Job drawing, mm, ordinate dimensions from the low corner. One solid piece. Round coordinates to 2 decimals unless told otherwise and drop trailing zeros. Write each loop counter-clockwise with the first axis right and the second up, starting at its lowest first coordinate (ties: lowest second). Pieces come first, ordered by that corner, then holes. Notation, with made-up numbers: (-2, 52) - (30, 52) arc R12 ccw to (30, 63) - close; hole circle Ø11 at (11, 2.25). An arc over 180 degrees is marked (long way). Write each question's results on one line, items separated by ' | '.
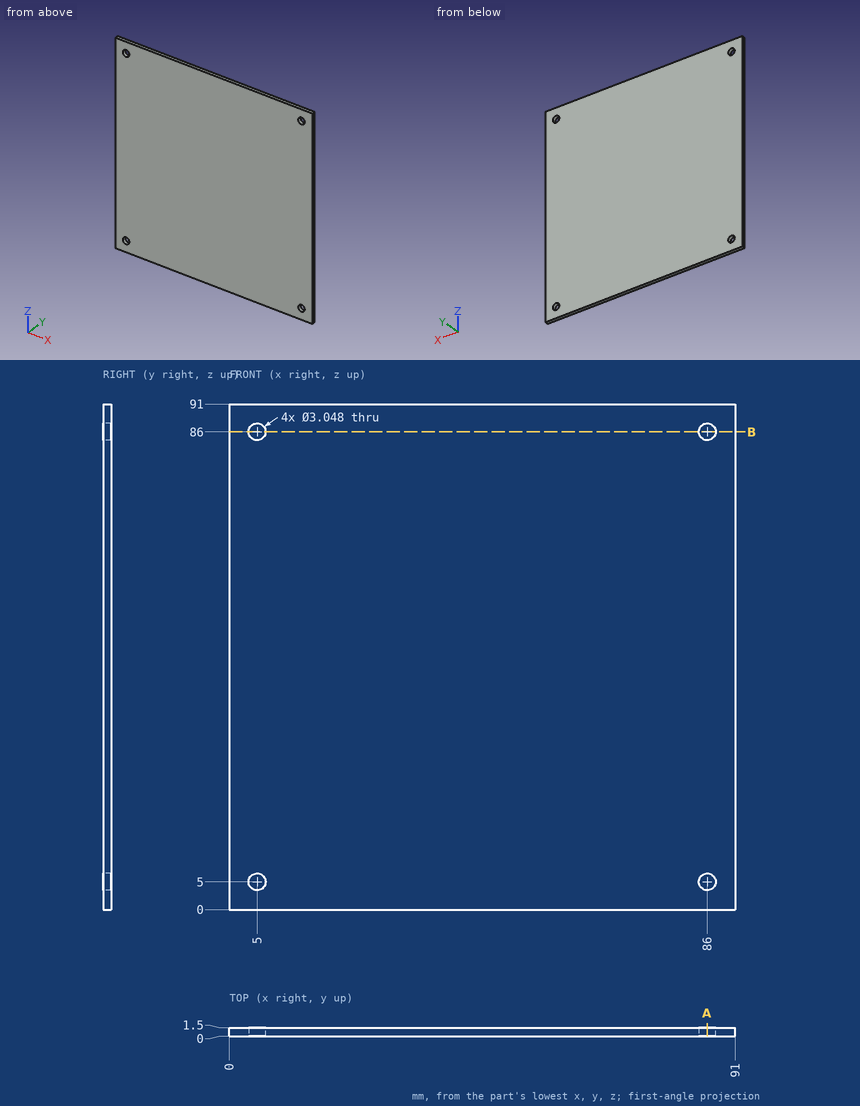
(1) Slice it at A-A, the plane x = 86. Write the cut outline in (y, z).
Worked answers:
outline: (0, 0) - (1.5, 0) - (1.5, 3.48) - (0, 3.48) - close; (0, 6.52) - (1.5, 6.52) - (1.5, 84.48) - (0, 84.48) - close; (0, 87.52) - (1.5, 87.52) - (1.5, 91) - (0, 91) - close
(2) Slice it at B-B, the plane z = 86. Write the cut outline in (x, y).
Worked answers:
outline: (0, 0) - (3.48, 0) - (3.48, 1.5) - (0, 1.5) - close; (6.52, 0) - (84.48, 0) - (84.48, 1.5) - (6.52, 1.5) - close; (87.52, 0) - (91, 0) - (91, 1.5) - (87.52, 1.5) - close
(3) Drill centre lines: probe 1 along Z at (x, y) = (5, 0.35); probe 2 along Z at (x, y) = (6, 1.1). Where is each one in solid material? Low to high. Write a range as [from, to].
Worked answers:
probe 1: z = [0, 3.48], [6.52, 84.48], [87.52, 91] | probe 2: z = [0, 3.85], [6.15, 84.85], [87.15, 91]
